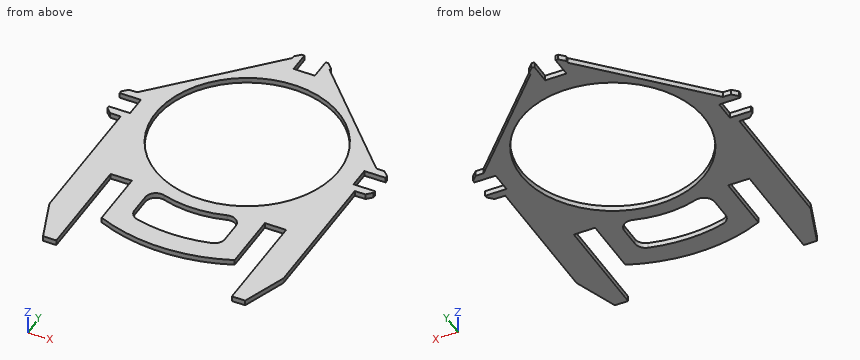
```python
from build123d import *

# Parameters (mm, degrees)
ESQUISSE1_R        = 172
BOSS_EXTRU_1_DEPTH = 10
CONG_1_R           = 20


with BuildPart() as part:
    # Esquisse1 → Boss.-Extru.1 (new body)
    with BuildSketch(Plane.XY):
        with BuildLine():
            Line((220, -297.575677416), (220, -228.230147001))
            Line((220, -228.230147001), (220, -35))
            Line((220, -35), (240, -35))
            Line((240, -35), (250, -25))
            Line((250, -25), (250, -20))
            Line((250, -20), (210, -20))
            Line((210, -20), (210, 20))
            Line((210, 20), (250, 20))
            Line((250, 20), (250, 25))
            Line((250, 25), (240, 35))
            Line((240, 35), (225, 35))
            Line((225, 35), (35, 235))
            Line((35, 235), (35, 240))
            Line((35, 240), (25, 250))
            Line((25, 250), (20, 250))
            Line((20, 250), (20, 210))
            Line((20, 210), (-20, 210))
            Line((-20, 210), (-20, 250))
            Line((-20, 250), (-25, 250))
            Line((-25, 250), (-35, 240))
            Line((-35, 240), (-35, 235))
            Line((-35, 235), (-225, 35))
            Line((-225, 35), (-240, 35))
            Line((-240, 35), (-250, 25))
            Line((-250, 25), (-250, 20))
            Line((-250, 20), (-210, 20))
            Line((-210, 20), (-210, -20))
            Line((-210, -20), (-250, -20))
            Line((-250, -20), (-250, -25))
            Line((-250, -25), (-240, -35))
            Line((-240, -35), (-220, -35))
            Line((-220, -35), (-220, -297.575677416))
            Line((-220, -297.575677416), (-190, -380))
            Line((-190, -380), (-165, -380))
            Line((-165, -380), (-165, -180))
            Line((-165, -180), (-125, -180))
            Line((-125, -180), (-125, -291.314263297))
            ThreePointArc((-125, -291.314263297), (0, -317), (125, -291.314263297))
            Line((125, -291.314263297), (125, -180))
            Line((125, -180), (165, -180))
            Line((165, -180), (165, -380))
            Line((165, -380), (190, -380))
            Line((190, -380), (220, -297.575677416))
        make_face()
        with BuildLine():
            Line((-85, -263.636112853), (-85, -180))
            ThreePointArc((-85, -180), (0, -199.060292374), (85, -180))
            Line((85, -180), (85, -263.636112853))
            ThreePointArc((85, -263.636112853), (0, -277), (-85, -263.636112853))
        make_face(mode=Mode.SUBTRACT)
        Circle(ESQUISSE1_R, mode=Mode.SUBTRACT)
    extrude(amount=BOSS_EXTRU_1_DEPTH)

    # Congé1
    cong_1_edges = [part.edges().sort_by_distance(p)[0] for p in [
        (-85, -263.636112853, 5),
        (85, -263.636112853, 5),
        (85, -180, 5),
        (-85, -180, 5),
    ]]
    fillet(cong_1_edges, radius=CONG_1_R)


solid = part.part
```
Can you work these out from the model? Positions are in its coordinate system, mm. Round coordinates to 2 decimals unless told otherwise and drop trailing zeros. Loops run counter-clockwise (first coordinate to the right, second up) from the corner with the lowest first, then second, coordinate; pieces in that order, holes last. Notation, with made-up numbers: M 35.5,-9.75 L 52.5,-9.75 A27 ccw 52.5,22.25 Z; hole C 51.25,18.5 d8. An arc over 180 degrees is marked long. Answer as a JSON object with one key per item and string values. Group by question number.
Q1. Imagine slicing it at C-C, the plane y = -255.5. Please give me the cut outline in (x, z), then the cut area to 3 significant figures.
Q2. Imagine slicing it at A-A, the plane y = 0. Please give me the cut outline in (x, z), then the cut area to 3 significant figures.
Q3. Imagine slicing it at B-B, the plane x = 0. Please give me the cut outline in (y, z), then the cut area to 3 significant figures.
Q4. Please list where these lines run through material, in increasing order: L1, parallel to X at y = -230.5, z = 2; L2, parallel to Y at x = 82, z = 0.5; L3, parallel to Y at x = -62, z = 0.5.
Q5. Imagine slicing it at D-D, the plane z = 7.5. Count the separate pieces of the cut face and the enclosed holes in it, then the cut area to 3 significant figures.
Q6. Will these pins go through, and if not, where does the flat tip stop? pin 1 (1 mm diameter, centred on x = 113.5, z = 7.5, fed in from -Y); pin 2 (1.5 mm diameter, centred on x = -48.5, z = 6.5, fed in from -Y); pin 3 (1.5 mm diameter, centred on x = 16.5, z = 2, fed in from +Y).
Findings:
{
 "1": {"outline": "M -220,0 L -165,0 L -165,10 L -220,10 Z; M -125,0 L -83.79,0 L -83.79,10 L -125,10 Z; M 83.79,0 L 125,0 L 125,10 L 83.79,10 Z; M 165,0 L 220,0 L 220,10 L 165,10 Z", "area": "1,920 mm2"},
 "2": {"outline": "M -210,0 L -172,0 L -172,10 L -210,10 Z; M 172,0 L 210,0 L 210,10 L 172,10 Z", "area": "760 mm2"},
 "3": {"outline": "M -317,0 L -277,0 L -277,10 L -317,10 Z; M -199.06,0 L -172,0 L -172,10 L -199.06,10 Z; M 172,0 L 210,0 L 210,10 L 172,10 Z", "area": "1,050 mm2"},
 "4": {"L1": "x = -220 to -165, -125 to -85, 85 to 125, 165 to 220", "L2": "y = -306.21 to -259.18, -198.66 to -151.2, 151.2 to 185.53", "L3": "y = -310.88 to -269.97, -189.42 to -160.44, 160.44 to 206.58"},
 "5": {"separate pieces": "1", "enclosed holes": "2", "area": "92,400 mm2"},
 "6": {"pin 1": "stops at y = -296.18", "pin 2": "stops at y = -313.38", "pin 3": "stops at y = 210"}
}
